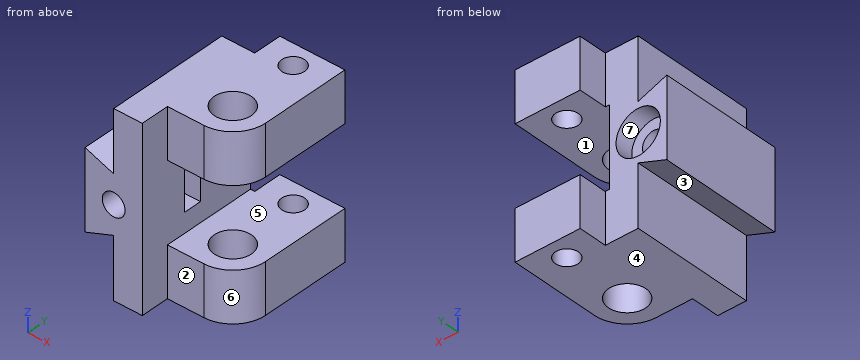
```python
from build123d import *

# Parameters (mm, degrees)
CROQUIS1_R                 = 2.6
SALIENTE_EXTRUIR1_DEPTH    = 25
CROQUIS2_W                 = 9.7
CROQUIS2_H                 = 11
CORTAR_EXTRUIR1_DEPTH      = 25
CROQUIS3_W                 = 4
CROQUIS3_H                 = 8
SALIENTE_EXTRUIR2_DEPTH    = 17.2
CORTAR_EXTRUIR2_DEPTH      = 1.25
CORTAR_EXTRUIR2_DEPTH_BACK = 1.25
CROQUIS5_R                 = 1.6
CORTAR_EXTRUIR3_DEPTH      = 34.25
SALIENTE_EXTRUIR3_DEPTH    = 17.2
SALIENTE_EXTRUIR4_REACH    = 31.505
CORTAR_EXTRUIR4_DEPTH      = 27.25
CORTAR_EXTRUIR4_DEPTH_BACK = 27.25
CROQUIS13_W                = 9.7
CROQUIS13_H                = 11
CROQUIS15_R                = 1.6
CORTAR_EXTRUIR6_DEPTH      = 27.25
CROQUIS16_W                = 0.6
CROQUIS16_H                = 3
CORTAR_EXTRUIR7_DEPTH      = 33
CROQUIS17_R                = 3.1
CORTAR_EXTRUIR8_DEPTH      = 2.5
CROQUIS18_W                = 9.1
CROQUIS18_H                = 7
SALIENTE_EXTRUIR5_DEPTH    = 1


with BuildPart() as part:
    # Croquis1 → Saliente-Extruir1 (new body)
    with BuildSketch(Plane.XY):
        with BuildLine():
            Line((-9.1, 8.6), (-5.1, 8.6))
            Line((-5.1, 8.6), (-5.1, 4.6))
            Line((-5.1, 4.6), (0, 4.6))
            ThreePointArc((0, 4.6), (4.6, 0), (0, -4.6))
            Line((0, -4.6), (-5.1, -4.6))
            Line((-5.1, -4.6), (-5.1, -8.6))
            Line((-5.1, -8.6), (-9.1, -8.6))
            Line((-9.1, -8.6), (-9.1, 8.6))
        make_face()
        Circle(CROQUIS1_R, mode=Mode.SUBTRACT)
    extrude(amount=SALIENTE_EXTRUIR1_DEPTH)

    # Croquis2 → Cortar-Extruir1 (cut)
    with BuildSketch(Plane(origin=(0, 4.6, 0), x_dir=(1, 0, 0), z_dir=(0, 1, 0))):
        with Locations((-0.25, -12.5)):
            Rectangle(CROQUIS2_W, CROQUIS2_H)
    extrude(amount=-CORTAR_EXTRUIR1_DEPTH, mode=Mode.SUBTRACT)

    # Croquis3 → Saliente-Extruir2 (add)
    with BuildSketch(Plane(origin=(0, 8.6, 0), x_dir=(1, 0, 0), z_dir=(0, 1, 0))):
        with Locations((-11.1, -12.5)):
            Rectangle(CROQUIS3_W, CROQUIS3_H)
    extrude(amount=-SALIENTE_EXTRUIR2_DEPTH)

    # Croquis4 → Cortar-Extruir2 (cut, two sides: drawn at the far end of the back side and taken through both)
    with BuildSketch(Plane(origin=(0, -0.6, 0), x_dir=(-1, 0, 0), z_dir=(0, -1, 0)).offset(-CORTAR_EXTRUIR2_DEPTH_BACK)):
        Polygon((7.01228676, -9.75), (5.1, -9.75), (5.1, -15.25), (7.01228676, -15.25), (10.68771324, -15.25), (12.275426481, -12.5), (10.68771324, -9.75), align=None)
    extrude(amount=CORTAR_EXTRUIR2_DEPTH + CORTAR_EXTRUIR2_DEPTH_BACK, mode=Mode.SUBTRACT)

    # Croquis5 → Cortar-Extruir3 (cut)
    with BuildSketch(Plane.XZ.offset(8.6)):
        with Locations(Location((-9.1, 12.5, 0), (0, 0, 270))):
            Circle(CROQUIS5_R)
    extrude(amount=-CORTAR_EXTRUIR3_DEPTH, mode=Mode.SUBTRACT)

    # Croquis6 → Saliente-Extruir3 (add)
    with BuildSketch(Plane.XZ.offset(8.6)):
        Polygon((-13.1, 18), (-9.1, 16.5), (-13.1, 16.5), align=None)
        Polygon((-13.1, 8.5), (-13.1, 7), (-9.1, 8.5), align=None)
    extrude(amount=-SALIENTE_EXTRUIR3_DEPTH)

    # Saliente-Extruir4: up to this face of the body (flat: up to its plane)
    saliente_extruir4_end = Plane(part.part.faces().sort_by_distance((-4.253300765, 0, 0))[0])
    # Croquis12 → Saliente-Extruir4 (add, up to the picked face)
    with BuildSketch(Plane.XY.offset(25), mode=Mode.PRIVATE) as saliente_extruir4_sk1:
        with BuildLine():
            Line((1.9, 11.6), (4.6, 11.6))
            Line((4.6, 11.6), (4.6, 0))
            Line((4.6, 0), (4, 0))
            ThreePointArc((4, 0), (2.828427125, 2.828427125), (0, 4))
            Line((0, 4), (0, 4.6))
            Line((0, 4.6), (-5.1, 4.6))
            Line((-5.1, 4.6), (-5.1, 11.6))
            Line((-5.1, 11.6), (1.9, 11.6))
        make_face()
    saliente_extruir4_tool1 = split(extrude(saliente_extruir4_sk1.sketch, amount=-SALIENTE_EXTRUIR4_REACH, mode=Mode.PRIVATE), bisect_by=saliente_extruir4_end, keep=Keep.BOTH, mode=Mode.PRIVATE)
    add(saliente_extruir4_tool1.solids().sort_by(Axis((0.135432, 7.547356, 25), (0, 0, -1)))[0])

    # Croquis13 → Cortar-Extruir4 (cut, two sides: drawn at the far end of the back side and taken through both)
    with BuildSketch(Plane.XZ.offset(-4.6).offset(-CORTAR_EXTRUIR4_DEPTH_BACK)):
        with Locations((-0.25, 12.5)):
            Rectangle(CROQUIS13_W, CROQUIS13_H)
    extrude(amount=CORTAR_EXTRUIR4_DEPTH + CORTAR_EXTRUIR4_DEPTH_BACK, mode=Mode.SUBTRACT)

    # Croquis15 → Cortar-Extruir6 (cut)
    with BuildSketch(Plane.XY.offset(25)):
        with Locations((0, 9.6)):
            Circle(CROQUIS15_R)
    extrude(amount=-CORTAR_EXTRUIR6_DEPTH, mode=Mode.SUBTRACT)

    # Croquis16 → Cortar-Extruir7 (cut)
    with BuildSketch(Plane.XY.offset(25)):
        with Locations((-4.8, 10.1)):
            Rectangle(CROQUIS16_W, CROQUIS16_H)
    extrude(amount=-CORTAR_EXTRUIR7_DEPTH, mode=Mode.SUBTRACT)

    # Croquis17 → Cortar-Extruir8 (cut)
    with BuildSketch(Plane(origin=(0, 8.6, 0), x_dir=(1, 0, 0), z_dir=(0, 1, 0))):
        with Locations(Location((-9.1, -12.5, 0), (0, 0, 270))):
            Circle(CROQUIS17_R)
    extrude(amount=-CORTAR_EXTRUIR8_DEPTH, mode=Mode.SUBTRACT)

    # Croquis18 → Saliente-Extruir5 (add)
    with BuildSketch(Plane(origin=(0, 11.6, 0), x_dir=(1, 0, 0), z_dir=(0, 1, 0))):
        with Locations((0.05, -21.5)):
            Rectangle(CROQUIS18_W, CROQUIS18_H)
        with Locations((0.05, -3.5)):
            Rectangle(CROQUIS18_W, CROQUIS18_H)
    extrude(amount=SALIENTE_EXTRUIR5_DEPTH)


solid = part.part
```
Part model, mm, in its own coordinate system. Face numbers are marked on the shaded views. A direction names the side the tool comes from. Coordinates: 2 decimals unless noted, no trailing zeros. Write each loop counter-clockwise with the first axis right and the second up, starting at its lowest first coordinate (ties: lowest second). Pieces come first, ordered by that corner, then holes.
Item 1: Probe line 1 (X direction, y = -4.75, z = 12.5); line 2 (Y direction, x = -5.25, z = 13.5); line 3 (Z direction, x = 3.5, y = 9.5). List the from-to ranges inside material, lowest first.
Item 2: Slice it at C-C (y = 9.6). Write the cut outline in (x, z).
Item 3: Mould opens along Z. For the marked faces 4, 5, 6 and 7 say: released by +Z, released by -Z, zero draft, split by the parting line, or undercut.
Item 4: Slice it at A-A (z = 21). Write the cut outline in (x, y), and give its area (3 significant figures).
Item 5: Which spindle directions (+Z, -Z, +X, -X, +Y, -Y) get a long thin tool onto all of the face, cutting with end or side? Do the marked faces 1, 2 and 3. Say none if no direction does.
Item 6: Pin check, flat tips, straight feed: pin 1 (2.5 mm diameter, centred on x = 0, y = 9.6, fed in from -Z); pin 2 (4.5 mm diameter, centred on y = 11.5, z = 21, fed in from -X); pin 3 (4.5 mm diameter, centred on x = -7, z = 18.5, fed in from +Y); pin 4 (4 mm diameter, centred on y = -3.5, z = 21, fed in from -X). Stop position of each tip, or through.
Item 7: Slice it at D-D (z = 13.25). Write the cut outline in (x, y).
Item 8: Slice it at B-B (x = -3.25). Write the cut outline in (y, z).
Results found:
1. line 1: x = -13.1 to -10.7, -7.5 to -5.1
1. line 2: y = -8.6 to -1.85, 0.65 to 8.6
1. line 3: z = 0 to 7, 18 to 25
2. outline: (-4.5, 0) - (-1.6, 0) - (-1.6, 7) - (-4.5, 7) - close; (-4.5, 18) - (-1.6, 18) - (-1.6, 25) - (-4.5, 25) - close; (1.6, 0) - (4.6, 0) - (4.6, 7) - (1.6, 7) - close; (1.6, 18) - (4.6, 18) - (4.6, 25) - (1.6, 25) - close
3. face 4: released by -Z
3. face 5: undercut
3. face 6: zero draft
3. face 7: undercut
4. outline: (-9.1, -8.6) - (-5.1, -8.6) - (-5.1, -4.6) - (0, -4.6) arc R4.6 ccw to (4.6, 0) - (4.6, 12.6) - (-4.5, 12.6) - (-4.5, 8.6) - (-9.1, 8.6) - close; hole circle Ø5.2 at (0, 0); hole circle Ø3.2 at (0, 9.6)
4. area: 199 mm2
5. face 1: +X, +Y, -Y
5. face 2: +Z, -Z, +X, -Y
5. face 3: -Z, +Y, -Y
6. pin 1: passes through
6. pin 2: stops at x = -4.5
6. pin 3: stops at y = 8.6
6. pin 4: stops at x = -9.1
7. outline: (-13.1, -8.6) - (-10.51, -8.6) - (-10.51, -1.85) - (-11.84, -1.85) - (-11.84, 0.65) - (-10.51, 0.65) - (-10.51, 6.1) - (-12.11, 6.1) - (-12.11, 8.6) - (-13.1, 8.6) - close; (-7.69, -8.6) - (-5.1, -8.6) - (-5.1, -1.85) - (-7.69, -1.85) - close; (-7.69, 0.65) - (-5.1, 0.65) - (-5.1, 8.6) - (-6.09, 8.6) - (-6.09, 6.1) - (-7.69, 6.1) - close
8. outline: (-4.6, 0) - (12.6, 0) - (12.6, 7) - (-4.6, 7) - close; (-4.6, 18) - (12.6, 18) - (12.6, 25) - (-4.6, 25) - close
